```python
from build123d import *

# Parameters (mm, degrees)
CORTE_EXTRUS_O1_DEPTH      = 10
CHANFRO3_SIZE              = 1.2
CORTE_EXTRUS_O2_DEPTH      = 33.865482391
CORTE_EXTRUS_O2_DEPTH_BACK = 33.865482391
ESBO_O5_R                  = 0.5


with BuildPart() as part:
    # Esboço2 → Revolução1 (revolve)
    with BuildSketch(Plane.XY, mode=Mode.PRIVATE) as revolu_o1_sk:
        Polygon((6, 0), (23, 0), (23, 0.5), (21, 1.352653961), (21, 3.352653961), (23, 4.205307923), (23, 4.705307923), (6, 4.705307923), align=None)
    revolve(revolu_o1_sk.sketch.rotate(Axis((0, 0, 0), (0, 1, 0)), 90), axis=Axis((0, 0, 0), (0, 1, 0)))

    # Esboço3 → Corte-extrusão1 (cut)
    with BuildSketch(Plane.XZ):
        with BuildLine():
            Line((23.115047023, 0.75), (23.115047023, -0.75))
            Line((23.115047023, -0.75), (22.384848004, -0.75))
            ThreePointArc((22.384848004, -0.75), (17.5, 0), (22.384848004, 0.75))
            Line((22.384848004, 0.75), (23.115047023, 0.75))
        make_face()
    extrude(amount=-CORTE_EXTRUS_O1_DEPTH, mode=Mode.SUBTRACT)

    # Chanfro3
    chanfro3_edges = [part.edges().sort_by_distance(p)[0] for p in [
        (0, 0, 6),
        (0, 4.705307923, 6),
    ]]
    chamfer(chanfro3_edges, length=CHANFRO3_SIZE)

    # Esboço5 → Corte-extrusão2 (cut, two sides: drawn at the far end of the back side and taken through both)
    with BuildSketch(Plane(origin=(0, 4.705307923, 0), x_dir=(1, 0, 0), z_dir=(0, 1, 0)).offset(-CORTE_EXTRUS_O2_DEPTH_BACK)):
        with Locations(Location((0, 13, 0), (0, 0, 270))):
            Circle(ESBO_O5_R)
        with Locations(Location((0, -13, 0), (0, 0, 270))):
            Circle(ESBO_O5_R)
        with Locations(Location((11.258330249, 6.5, 0), (0, 0, 270))):
            Circle(ESBO_O5_R)
        with Locations(Location((-11.258330249, -6.5, 0), (0, 0, 270))):
            Circle(ESBO_O5_R)
        with Locations(Location((11.258330249, -6.5, 0), (0, 0, 270))):
            Circle(ESBO_O5_R)
        with Locations(Location((-11.258330249, 6.5, 0), (0, 0, 270))):
            Circle(ESBO_O5_R)
    extrude(amount=CORTE_EXTRUS_O2_DEPTH + CORTE_EXTRUS_O2_DEPTH_BACK, mode=Mode.SUBTRACT)


solid = part.part
```
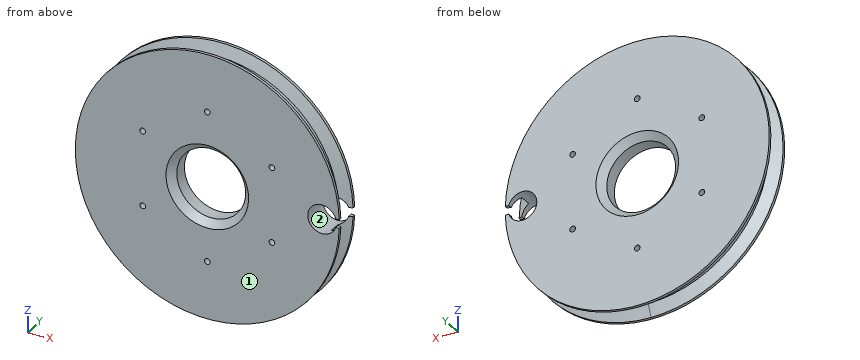
The listing builds one solid part. Answer for the finished solid, in the listing's coordinates (mm). Face numbers are marked on the shaded views. Coordinates: 2 decimals unless noted, no trailing zeros. Loops run counter-clockwise (first coordinate to the right, second up) from the corner with the lowest first, then second, coordinate; pieces in that order, holes last. Notation, with made-up numbers: (56.5, -4) -> (84.5, -4) arc R29 ccw to (84.5, 27) -> close; hole circle Ø3 at (2.5, 40.5). An arc over 180 degrees is marked (long way). Return JSON: item names as keys, results as strings. Group by question number.
(1) Given pin 1 Ø2 at (y, z) = (1, -14.5) entering from +X, flat-ended and moving along its own axis, determine where the tip first touches the part or whether it passes through.
(2) Find the intervals of material crossed by probe 1 along X at (y, z) = (2.9, -6.5); probe 2 along Z at (x, y) = (-1, 2.15); probe 3 along X at (y, z) = (1.4, 0), in increasing order. Write a range as from..to.
(3) A cutting plane is placed at A-A on z = 0. Write down the section's boundary in (x, y), and give its area (3 significant figures).
(4) A cutting plane is placed at B-B on y = 2.8. Write down the section's boundary in (x, z).
(5) Determine the mould class of the marked faces 1 and 2 for opening direction Z: released by +Z, released by -Z, zero draft, split by the parting line, or undercut.
The answers:
{
 "1": {"pin 1": "stops at x = 18.52"},
 "2": {"probe 1": "x = -19.97..-11.76, -10.76..10.76, 11.76..19.97", "probe 2": "z = -20.98..-5.92, 5.92..20.98", "probe 3": "x = -21..-6, 6..17.5"},
 "3": {"outline": "(-23, 0) -> (-7.2, 0) -> (-6, 1.2) -> (-6, 3.51) -> (-7.2, 4.71) -> (-23, 4.71) -> (-23, 4.21) -> (-21, 3.35) -> (-21, 1.35) -> (-23, 0.5) -> close; (6, 1.2) -> (7.2, 0) -> (17.5, 0) -> (17.5, 4.71) -> (7.2, 4.71) -> (6, 3.51) -> close", "area": "126 mm^2"},
 "4": {"outline": "(20.87, -2.34) arc R2.5 cw (long way) to (20.87, 2.34) arc R21 ccw (long way) to start; hole circle Ø1 at (-11.26, -6.5); hole circle Ø1 at (-11.26, 6.5); hole circle Ø12 at (0, 0); hole circle Ø1 at (0, -13); hole circle Ø1 at (0, 13); hole circle Ø1 at (11.26, -6.5); hole circle Ø1 at (11.26, 6.5)"},
 "5": {"face 1": "zero draft", "face 2": "undercut"}
}
